Geometry check sheet. Reference: the model listing, model coordinates, mm. Face numbers are marked on the shaded views. Give positions to 0.01 mm unless a question says otherwise; leave off trailing zeros. Write each loop counter-clockwise with the first axis right and the second up, starting at its lowest first coordinate (ties: lowest second). Pieces come first, ordered by that corner, then holes.
(1) Cross-section at C-C (z = 17). Record the boundary of the cut face in (x, y), and give its area (3 significant figures).
(2) Thickness scan on line 1 along X through (y, z) = (15, 22.5); line 2 along Z through (x, y) = (71, 0) (3 decimals); line 3 along Y through (x, z) = (3, 31). Record the ranges inside material, lowest first.
(3) Cross-section at D-D (z = 31.75). Record the boundary of the cut face in (x, y), and give its area (3 significant figures).
(4) Cross-section at A-A (y = 0). Record the boundary of the cut face in (x, z) (3 decimals), and give its area (3 significant figures).
(5) Depth check by flat-ended pin: P1, Ø6, axis at x = 53.5, y = -32.5, coming from the -Z side; P2, Ø4, axis at x = 23, y = -19.5, coming from the +Z side; P3, Ø12, axis at x = 8.5, y = 24, coming from the -Z side. Enter the tip coordinate at first touch or a pass-through.
(6) Mould release check, pull along X, two halves, no side actions. Record for the marked faces 1, 2 and 3: +X half, -X half, draft (parallel to the pull), parting line (faces both ways), or undercut.
```python
from build123d import *

# Parameters (mm, degrees)
F0_R          = 3.96875
F1_DEPTH      = 76.2
F4_DEPTH      = 26.543
F4_DEPTH_BACK = 26.543


with BuildPart() as f1:
    # F0 (on Right) → F1 (new body)
    with BuildSketch(Plane.YZ):
        with BuildLine():
            Line((-53.975, 4.7625), (-53.975, 0))
            ThreePointArc((-53.975, 0), (0, 6.985), (53.975, 0))
            Line((53.975, 0), (53.975, 4.7625))
            Line((53.975, 4.7625), (3.7789439849, 37.5375718687))
            ThreePointArc((3.7789439849, 37.5375718687), (0, 38.6620478714), (-3.7789439849, 37.5375718687))
            Line((-3.7789439849, 37.5375718687), (-53.975, 4.7625))
        make_face()
        with Locations((0, 31.75)):
            Circle(F0_R, mode=Mode.SUBTRACT)
    extrude(amount=F1_DEPTH)

    # F3 (on offset) → F4 (cut, two sides)
    with BuildSketch(Plane(origin=(38.1, 0, 0), x_dir=(0, -1, 0), z_dir=(-1, 0, 0))) as f4_sk:
        with BuildLine():
            ThreePointArc((3.7789439849, 37.5375718687), (0, 38.6620478714), (-3.7789439849, 37.5375718687))
            Line((-3.7789439849, 37.5375718687), (-53.975, 4.7625))
            ThreePointArc((-53.975, 4.7625), (0, 11.7472640284), (53.975, 4.7625))
            Line((53.975, 4.7625), (3.7789439849, 37.5375718687))
        make_face()
    extrude(amount=F4_DEPTH, mode=Mode.SUBTRACT)
    extrude(f4_sk.sketch, amount=-F4_DEPTH_BACK, mode=Mode.SUBTRACT)


solid = f1.part
```
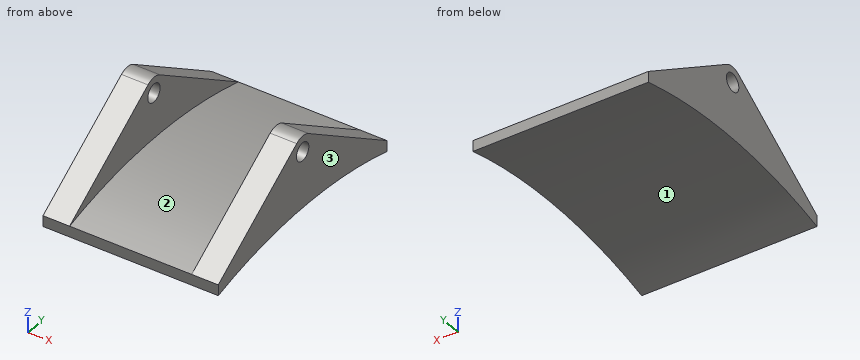
Reply:
1. outline: (0, -35.23) - (11.56, -35.23) - (11.56, 35.23) - (0, 35.23) - close; (64.64, -35.23) - (76.2, -35.23) - (76.2, 35.23) - (64.64, 35.23) - close
1. area: 1,630 mm2
2. line 1: x = 0 to 11.56, 64.64 to 76.2
2. line 2: z = 6.985 to 27.781, 35.719 to 38.662
2. line 3: y = -13.79 to -3.9, 3.9 to 13.79
3. outline: (0, -12.64) - (11.56, -12.64) - (11.56, -3.97) - (0, -3.97) - close; (0, 3.97) - (11.56, 3.97) - (11.56, 12.64) - (0, 12.64) - close; (64.64, -12.64) - (76.2, -12.64) - (76.2, -3.97) - (64.64, -3.97) - close; (64.64, 3.97) - (76.2, 3.97) - (76.2, 12.64) - (64.64, 12.64) - close
3. area: 401 mm2
4. outline: (0, 6.985) - (76.2, 6.985) - (76.2, 27.781) - (64.643, 27.781) - (64.643, 11.747) - (11.557, 11.747) - (11.557, 27.781) - (0, 27.781) - close; (0, 35.719) - (11.557, 35.719) - (11.557, 38.662) - (0, 38.662) - close; (64.643, 35.719) - (76.2, 35.719) - (76.2, 38.662) - (64.643, 38.662) - close
4. area: 802 mm2
5. P1: stops at z = 3.99
5. P2: stops at z = 11.02
5. P3: stops at z = 4.85
6. face 1: draft
6. face 2: undercut
6. face 3: +X half
